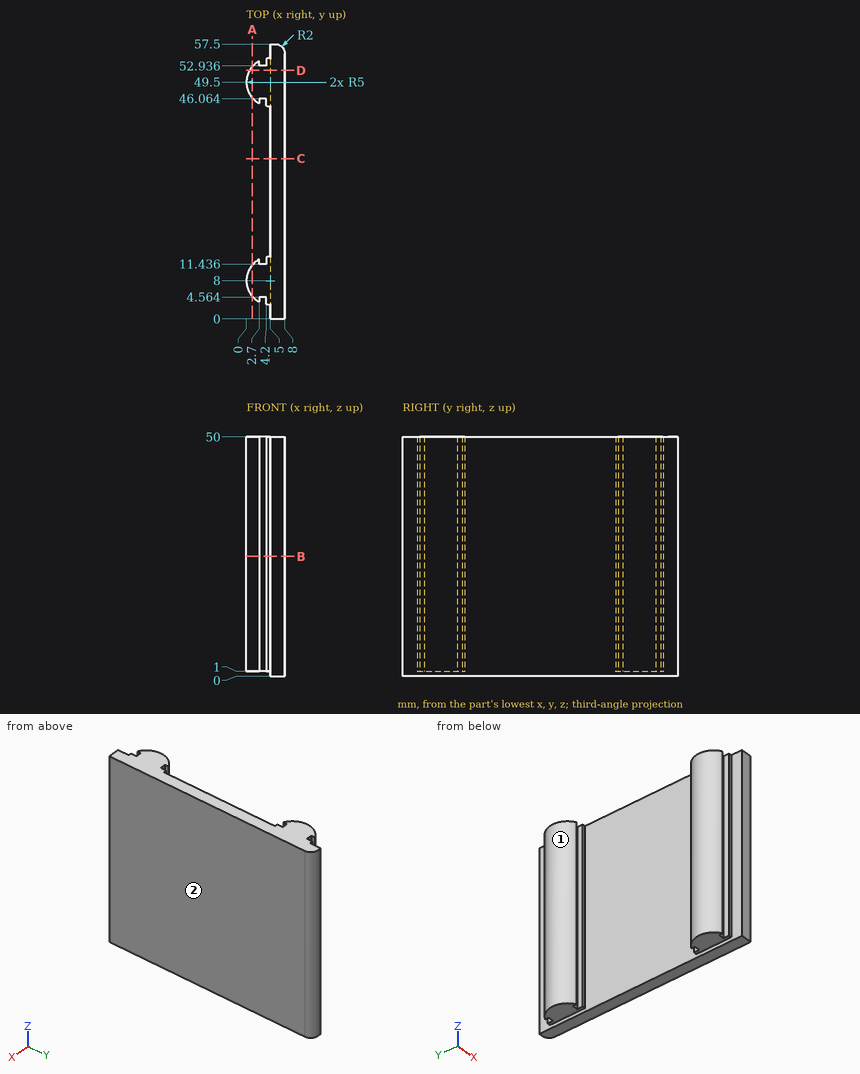
Could you check a few things on this drawing? It's one solid part, dimensions in mm from its lowest x, y, z. Give positions to 0.01 mm unless a question says otherwise; leave off trailing zeros. Write each loop counter-clockwise with the first axis right and the second up, starting at its lowest first coordinate (ties: lowest second). Pieces come first, ordered by that corner, then holes. Notation, with made-up numbers: (62.5, -35) -> (97.5, -35) arc R26 cw to (97.5, 3) -> close; hole circle Ø10 at (-4, 80.5). An arc over 180 degrees is marked (long way). Answer as CSV lines item,"result". Start each with the question number.
(1) If we section it at D-D, the plane y = 52: Write out the boundary of the cut face in (x, z).
(2) If we section it at C-C, the plane y = 33.5: Write out the boundary of the cut face in (x, z), and give its area (3 significant figures).
(3) Please list where these lines run through material, in increasing order: line 1 (Y direction, x = 3.5, z = 18.5) (1 decimal); line 2 (Y direction, x = 4.25, z = 41); line 3 (X direction, y = 14, z = 41.5).
(4) If we section it at A-A, the plane x = 1.25: Write out the boundary of the cut face in (y, z), and give its area (3 significant figures).
(5) If we section it at B-B, the plane z = 25: Write out the boundary of the cut face in (x, y) (1 decimal).
(6) I'm going to push flat-ended pins straight in: pin 1 Ø1.6 at (y, z) = (12.5, 28) entering from -X; pin 2 Ø1.2 at (y, z) = (4, 33.5) entering from -X (1 decimal); pin 3 Ø3 at (x, z) = (1, 20) entering from -Y. Where does each tip first touch, or does it pass through?
(7) If we mould it in two halves opening along Y, with no side actions, what happens to the marked faces 1 and 2? For each: +Y half, -Y half, draft (parallel to the pull), parting line (faces both ways), or undercut.
Answer list:
1,outline,"(0.67, 1) -> (5, 1) -> (5, 0) -> (8, 0) -> (8, 50) -> (0.67, 50) -> close"
2,outline,"(5, 0) -> (8, 0) -> (8, 50) -> (5, 50) -> close"
2,area,"150 mm^2"
3,line 1,"4.6 to 11.4, 46.1 to 52.9"
3,line 2,"3.06 to 12.94, 44.56 to 54.44"
3,line 3,"5 to 8"
4,outline,"(4.69, 1) -> (11.31, 1) -> (11.31, 50) -> (4.69, 50) -> close; (46.19, 1) -> (52.81, 1) -> (52.81, 50) -> (46.19, 50) -> close"
4,area,"648 mm^2"
5,outline,"(2.7, 3.6) -> (2.7, 4.6) -> (4.2, 4.6) -> (4.2, 3.1) arc R5 ccw to (5, 3) -> (5, 0) -> (8, 0) -> (8, 55.5) arc R2 ccw to (6, 57.5) -> (5, 57.5) -> (5, 54.5) arc R5 ccw to (4.2, 54.4) -> (4.2, 52.9) -> (2.7, 52.9) -> (2.7, 53.9) arc R5 ccw to (2.7, 45.1) -> (2.7, 46.1) -> (4.2, 46.1) -> (4.2, 44.6) arc R5 ccw to (5, 44.5) -> (5, 13) arc R5 ccw to (4.2, 12.9) -> (4.2, 11.4) -> (2.7, 11.4) -> (2.7, 12.4) arc R5 ccw to start"
6,pin 1,"x = 1.64"
6,pin 2,"x = 1.3"
6,pin 3,"y = 3.67"
7,face 1,"undercut"
7,face 2,"draft"
